```python
from build123d import *

# Parameters (mm, degrees)
BOSS_EXTRUDE1_DEPTH = 8.89
SKETCH2_W           = 35.56
SKETCH2_H           = 17.78
BOSS_EXTRUDE2_DEPTH = 22.86
SKETCH4_W           = 35.56
SKETCH4_H           = 7.112
CUT_EXTRUDE2_DEPTH  = 27.94
SKETCH5_W           = 35.56
SKETCH5_H           = 4.445
CUT_EXTRUDE3_DEPTH  = 7.62
SKETCH6_R           = 3.175
CUT_EXTRUDE4_DEPTH  = 6.35
FILLET1_R           = 12.7
FILLET2_R           = 3.175
FILLET3_R           = 3.175
FILLET6_R           = 2.54
BOSS_EXTRUDE5_DEPTH = 5.08
SKETCH14_R          = 3.175
CUT_EXTRUDE8_DEPTH  = 9.525
FILLET7_R           = 2.54


with BuildPart() as part:
    # Sketch1 → Boss-Extrude1 (new body)
    with BuildSketch(Plane(origin=(0, 0, 0), x_dir=(1, 0, 0), z_dir=(0, 1, 0))):
        Polygon((12.7, 7.62), (12.7, 0), (3.81, 0), (3.81, -8.89), (0, -8.89), (0, 0), (0, 25.4), (35.56, 25.4), (35.56, 0), (35.56, -8.89), (31.75, -8.89), (31.75, 0), (22.86, 0), (22.86, 7.62), align=None)
    extrude(amount=BOSS_EXTRUDE1_DEPTH)

    # Sketch2 → Boss-Extrude2 (add)
    with BuildSketch(Plane(origin=(0, 8.89, 0), x_dir=(1, 0, 0), z_dir=(0, 1, 0))):
        with Locations((17.78, 16.51)):
            Rectangle(SKETCH2_W, SKETCH2_H)
    extrude(amount=BOSS_EXTRUDE2_DEPTH)

    # Sketch4 → Cut-Extrude2 (cut)
    with BuildSketch(Plane(origin=(0, 31.75, 0), x_dir=(1, 0, 0), z_dir=(0, 1, 0))):
        with Locations((17.78, 15.621)):
            Rectangle(SKETCH4_W, SKETCH4_H)
    extrude(amount=-CUT_EXTRUDE2_DEPTH, mode=Mode.SUBTRACT)

    # Sketch5 → Cut-Extrude3 (cut)
    with BuildSketch(Plane(origin=(0, 31.75, 0), x_dir=(1, 0, 0), z_dir=(0, 1, 0))):
        with Locations((17.78, 9.8425)):
            Rectangle(SKETCH5_W, SKETCH5_H)
    extrude(amount=-CUT_EXTRUDE3_DEPTH, mode=Mode.SUBTRACT)

    # Sketch6 → Cut-Extrude4 (cut)
    with BuildSketch(Plane(origin=(0, 0, -25.4), x_dir=(-1, 0, 0), z_dir=(0, 0, -1))):
        with Locations((-17.78, 27.305)):
            Circle(SKETCH6_R)
    extrude(amount=-CUT_EXTRUDE4_DEPTH, mode=Mode.SUBTRACT)

    # Fillet1
    fillet1_edges = [part.edges().sort_by_distance(p)[0] for p in [
        (0, 31.75, -22.2885),
        (35.56, 31.75, -22.2885),
    ]]
    fillet(fillet1_edges, radius=FILLET1_R)

    # Fillet2
    fillet2_edges = [part.edges().sort_by_distance(p)[0] for p in [
        (0, 24.13, -9.8425),
        (35.56, 24.13, -9.8425),
    ]]
    fillet(fillet2_edges, radius=FILLET2_R)

    # Fillet3
    fillet3_edges = [part.edges().sort_by_distance(p)[0] for p in [
        (17.78, 0, -7.62),
    ]]
    fillet(fillet3_edges, radius=FILLET3_R)

    # Fillet6
    fillet6_edges = [part.edges().sort_by_distance(p)[0] for p in [
        (3.81, 0, 4.445),
        (31.75, 0, 4.445),
        (17.78, 3.81, -19.177),
        (17.78, 3.81, -12.065),
    ]]
    fillet(fillet6_edges, radius=FILLET6_R)

    # Sketch13 → Boss-Extrude5 (add)
    with BuildSketch(Plane(origin=(0, 8.89, 0), x_dir=(1, 0, 0), z_dir=(0, 1, 0))):
        Polygon((3.81, 0), (0, 0), (0, 7.62), (12.7, 7.62), (12.7, 0), align=None)
        Polygon((35.56, 7.62), (22.86, 7.62), (22.86, 0), (31.75, 0), (35.56, 0), align=None)
    extrude(amount=BOSS_EXTRUDE5_DEPTH)

    # Sketch14 → Cut-Extrude8 (cut)
    with BuildSketch(Plane.XY):
        with Locations((8.255, 6.985)):
            Circle(SKETCH14_R)
        with Locations((27.305, 6.985)):
            Circle(SKETCH14_R)
    extrude(amount=-CUT_EXTRUDE8_DEPTH, mode=Mode.SUBTRACT)

    # Fillet7
    fillet7_edges = [part.edges().sort_by_distance(p)[0] for p in [
        (6.35, 13.97, 0),
        (6.35, 13.97, -7.62),
        (29.21, 13.97, 0),
        (29.21, 13.97, -7.62),
    ]]
    fillet(fillet7_edges, radius=FILLET7_R)


solid = part.part
```
CAD build for the part. Positions are in the model's coordinates, mm. A direction names the side the tool comes from. Give positions to 0.01 mm unless a question says otherwise; leave off trailing zeros. Write each loop counter-clockwise with the first axis right and the second up, starting at its lowest first coordinate (ties: lowest second). Pieces come first, ordered by that corner, then holes. Notation, with made-up numbers: (19.5, -27.75) -> (48.5, -27.75) arc R16 cw to (48.5, 1.25) -> close; hole circle Ø10 at (72, 20.5). An arc over 180 degrees is marked (long way). Write each question's results on one line, items separated by ' | '.
1. Wall check: probe 1 along Z at (x, y) = (34.5, 7) (3 decimals); probe 2 along Y at (x, z) = (17.78, -23.25); probe 3 along Z at (x, y) = (14, 11.5) (3 decimals). Give the ranges that are in metal, low to high. Write a range as [from, to].
Geometry check:
probe 1: [-25.4, -19.177], [-12.065, 8.89] | probe 2: [0, 24.13], [30.48, 31.75] | probe 3: [-25.4, -19.177], [-12.065, -7.62]
2. Cut at C-C, the plane y = 18. Write the cut outline in (x, z) (3 decimals).
Geometry check:
outline: (0, -25.4) -> (35.56, -25.4) -> (35.56, -19.177) -> (0, -19.177) -> close; (0, -12.065) -> (35.56, -12.065) -> (35.56, -7.62) -> (0, -7.62) -> close
3. Cut at B-B, the plane z = -2. Write the cut outline in (x, y) (3 decimals).
Geometry check:
outline: (0, 0) -> (12.7, 0) -> (12.7, 13.912) -> (0, 13.912) -> close; (22.86, 0) -> (35.56, 0) -> (35.56, 13.912) -> (22.86, 13.912) -> close; hole circle Ø6.35 at (8.255, 6.985); hole circle Ø6.35 at (27.305, 6.985)
4. Which spindle directions (+Z, -Z, +X, -X, +Y, -Y) get a long thin tool onto all of the face, cutting with end or side? Do faces 4 (the cylindrical face through (34.61, 23.22, -9.87)), 5 (the cylindrical face through (32.514, 0.724, 4.383)), 6 (the flat face through (6, 13.97, -4)), 7 (the flat face through (27, 7, -9.525)). Say none if no direction does.
Geometry check:
face 4: +Z, +X, +Y | face 5: +Z, -Y | face 6: +Z, +X, -X, +Y | face 7: +Z
5. Cut at A-A, the plane x = 17.78. Write the cut outline in (y, z) (3 decimals), then the cut area to 3 significant figures.
Geometry check:
outline: (0, -25.4) -> (24.13, -25.4) -> (24.13, -19.177) -> (6.35, -19.177) arc R2.54 cw to (3.81, -16.637) -> (3.81, -14.605) arc R2.54 cw to (6.35, -12.065) -> (24.13, -12.065) -> (24.13, -7.62) -> (3.175, -7.62) arc R3.175 ccw to (0, -10.795) -> close; (30.48, -25.4) -> (31.75, -25.4) -> (31.75, -19.177) -> (30.48, -19.177) -> close | area: 293 mm²
6. Two-plate mould, pull along X, no slides. Class faces 1 (the cylindrical face through (29.121, 14.734, -6.896)), 2 (the flat face through (35.56, 8, -8)), 3 (the flat face through (29, 4, 0)): pulls with the +X half, pulls with the -X half, needs draft (parallel to the pull), parting line crosses it, or undercut.
Geometry check:
face 1: needs draft | face 2: pulls with the +X half | face 3: undercut
7. Drop flat-ended pins along their axis: P1, Ø2, axis at x = 17.5, z = -5, coming from the -Y side; P2, Ø1.9, axis at x = 2.5, z = 5.5, coming from the +Y side; P3, Ø3, axis at x = 28, y = 7, coming from the +Z side (3 decimals); P4, Ø7.5, axis at x = 27.305, y = 6.985, coming from the +Z side. Give the stop position or say it passes through.
Geometry check:
P1: through | P2: y = 8.89 | P3: z = -9.525 | P4: z = 0
8. Cut at D-D, the plane z = -9. Write the cut outline in (x, y) (3 decimals), then the cut area to 3 significant figures.
Geometry check:
outline: (0, 0) -> (12.7, 0) -> (12.7, 0.556) -> (22.86, 0.556) -> (22.86, 0) -> (35.56, 0) -> (35.56, 20.955) arc R3.175 ccw to (32.385, 24.13) -> (3.175, 24.13) arc R3.175 ccw to (0, 20.955) -> close; hole circle Ø6.35 at (8.255, 6.985); hole circle Ø6.35 at (27.305, 6.985) | area: 785 mm²
